The figure shows three views and two pictorial views of one solid part (mm, origin at its lowest corner). Answer the questions. A direction names the side the tool comes from. Round coordinates to 2 decimals unless told otherwise and drop trailing zeros. Order: outer loops, then holes, each group sorted by start corner. A loop starts at its lowest first (then second) coordinate and runs counter-clockwise, first axis right, second up.
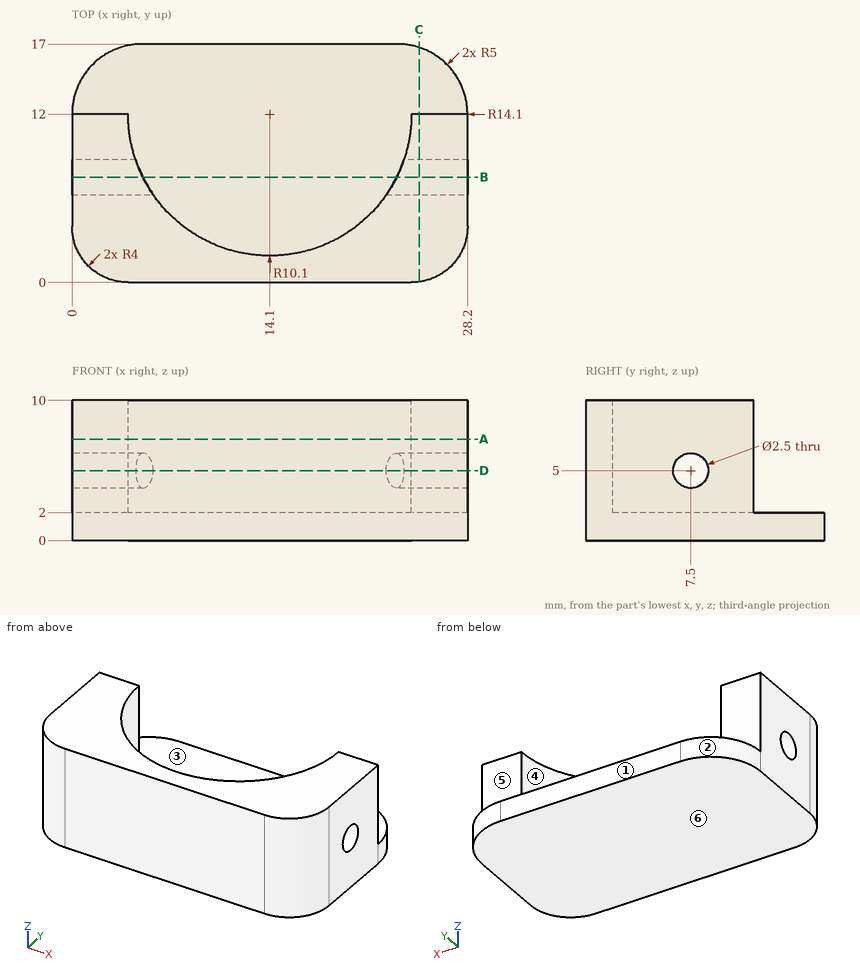
Item 1: A tool of negligible diameter and unlimited length cuts with its end or side. For the marked faces 5 and 6, from which of +Z, -Z, +X, -X, +Y, -Y can it reach the whole face along a straight path? Write none if from no direction.
Item 2: Find section D-D (z = 5). Write down the section's boundary in (x, y).
Item 3: For a pull along X with two mould halves and no side action, classify the marked faces 1, 2, 3 and 4 as released by +X, released by -X, zero draft, split by the parting line, or undercut.
Item 4: Find the intervals of material crossed by line 1 along Z through (x, y) = (1.35, 7.5); line 2 along Z through (x, y) = (18.75, 4.5); line 3 along X through (y, z) = (10.25, 6), in increasing order.
Item 5: Given pin 1 (2 mm diameter, centred on x = 1.5, z = 5, fed in from +Y); pin 2 (1.5 mm diameter, centred on x = 24.5, y = 9.5, fed in from -Z); pin 3 (5 mm diameter, centred on x = 7.5, y = 9.5, fed in from +Z), each flat-ended and moving along its own axis, determine where each tip first touches the part or whether it passes through.
Item 6: Find section B-B (y = 7.5). Write down the section's boundary in (x, z).
Item 7: Find section C-C (x = 24.75). Write down the section's boundary in (y, z), plus the area to 3 significant figures.
Item 8: Find section A-A (z = 7.25). Write down the section's boundary in (x, y), plus the area to 3 significant figures.
Model answer:
1. face 5: +Z, +X, -X, +Y
1. face 6: -Z, +X, -X, +Y, -Y
2. outline: (0, 4) arc R4 ccw to (4, 0) - (24.2, 0) arc R4 ccw to (28.2, 4) - (28.2, 6.25) - (22.4, 6.25) arc R10.1 cw to (5.8, 6.25) - (0, 6.25) - close; (0, 8.75) - (4.54, 8.75) arc R10.1 cw to (4, 12) - (0, 12) - close; (23.66, 8.75) - (28.2, 8.75) - (28.2, 12) - (24.2, 12) arc R10.1 cw to start
3. face 1: zero draft
3. face 2: released by -X
3. face 3: undercut
3. face 4: undercut
4. line 1: z = 0 to 3.75, 6.25 to 10
4. line 2: z = 0 to 2
4. line 3: x = 0 to 4.15, 24.05 to 28.2
5. pin 1: stops at y = 12
5. pin 2: stops at z = 0
5. pin 3: stops at z = 2
6. outline: (0, 0) - (28.2, 0) - (28.2, 3.75) - (23.14, 3.75) - (23.14, 2) - (5.06, 2) - (5.06, 3.75) - (0, 3.75) - close; (0, 6.25) - (5.06, 6.25) - (5.06, 10) - (0, 10) - close; (23.14, 6.25) - (28.2, 6.25) - (28.2, 10) - (23.14, 10) - close
7. outline: (0.04, 0) - (16.75, 0) - (16.75, 2) - (12, 2) - (12, 10) - (0.04, 10) - close; hole circle Ø2.5 at (7.5, 5)
7. area: 124 mm2
8. outline: (0, 4) arc R4 ccw to (4, 0) - (24.2, 0) arc R4 ccw to (28.2, 4) - (28.2, 12) - (24.2, 12) arc R10.1 cw to (4, 12) - (0, 12) - close
8. area: 171 mm2
